For this review, take the finished solid that the model builds, in its own axes (mm). A direction names the side the tool comes from. Give positions to 0.01 mm unless a question says otherwise; leave off trailing zeros. Loops run counter-clockwise (first coordinate to the right, second up) from the corner with the lowest first, then second, coordinate; pieces in that order, holes last. Notation, with made-up numbers: (69.5, 73) - (121.5, 73) arc R18 ccw to (121.5, 94) - close; hole circle Ø4 at (62.25, 69.25). An arc over 180 degrees is marked (long way). Put each result on its own line as item: value.
from build123d import *

# Parameters (mm, degrees)
F1_DEPTH = 4
F3_DEPTH = 0.8


with BuildPart() as f1:
    # F0 (on Top) → F1 (new body)
    with BuildSketch(Plane.XY):
        Polygon((-9.1288570138, -20.6640837675), (-18.5707826287, -20.6640837675), (-18.5707826287, -32.6640837675), (6.4292173713, -32.6640837675), (6.4292173713, -20.6640837675), (-8.1288570138, -20.6640837675), (-11.2707826287, -22.8640837675), (4.2292173713, -22.8640837675), (4.2292173713, -30.4640837675), (-16.3707826287, -30.4640837675), (-16.3707826287, -22.8640837675), (-12.2707826287, -22.8640837675), align=None)
    extrude(amount=F1_DEPTH)

    # F2 (on face) → F3 (join)
    with BuildSketch(Plane.XY.offset(4)):
        with BuildLine():
            ThreePointArc((-7.2837039026, -27.5826807615), (-9.0353563223, -29.6788503531), (-11.6517702118, -30.4640837675))
            Line((-11.6517702118, -30.4640837675), (4.2292173713, -30.4640837675))
            Line((4.2292173713, -30.4640837675), (4.2292173713, -25.1570476435))
            Line((4.2292173713, -25.1570476435), (-3.6065624964, -25.1570476435))
            ThreePointArc((-3.6065624964, -25.1570476435), (-5.8091215163, -25.8180756813), (-7.2837039026, -27.5826807615))
        make_face()
    extrude(amount=-F3_DEPTH)


solid = f1.part
1) For faces 4 (the face through (-16.371, -27, 2)), 5 (the face through (-2, -28, 3.2)), 6 (the face through (-1, -20.664, 2)), list the 3-axis set-ups (+Z, -Z, +X, -X, +Y, -Y) from which the entire face can be reached by the end or side of a thin tool; tool diameter is ignored.
Geometry check:
face 4: +Z, -Z
face 5: -Z
face 6: +Z, -Z, +X, -X, +Y
2) Take a section at B-B on y = -24. State the section outline as (x, z) points, and give its area (3 significant figures).
Geometry check:
outline: (-18.57, 0) - (-16.37, 0) - (-16.37, 4) - (-18.57, 4) - close; (4.23, 0) - (6.43, 0) - (6.43, 4) - (4.23, 4) - close
area: 17.6 mm²
3) Take a section at C-C on x = -14. State the section outline as (y, z) points, and give its area (3 significant figures).
Geometry check:
outline: (-32.66, 0) - (-30.46, 0) - (-30.46, 4) - (-32.66, 4) - close; (-22.86, 0) - (-20.66, 0) - (-20.66, 4) - (-22.86, 4) - close
area: 17.6 mm²
4) Insertion check: pin 1 Ø4 at (x, y) = (-0.5, -26.5) entering from -Z. The pin has a flat end and moves straight along its axis. Give the tip position at first contact, or say it passes through.
Geometry check:
pin 1: stops at z = 3.2
5) Take a section at A-A on x = 0.75. State the section outline as (y, z) points.
Geometry check:
outline: (-32.66, 0) - (-30.46, 0) - (-30.46, 3.2) - (-25.16, 3.2) - (-25.16, 4) - (-32.66, 4) - close; (-22.86, 0) - (-20.66, 0) - (-20.66, 4) - (-22.86, 4) - close
6) Wall thickness on line 1 (X direction, y = -26, z = 1.4); line 2 (Y direction, x = -0.25, z = 3.75); line 3 (Y direction, x = -5.25, z = 2.2): over which ranges is each line inside the solid? List them lowest first.
Geometry check:
line 1: x = -18.57 to -16.37, 4.23 to 6.43
line 2: y = -32.66 to -25.16, -22.86 to -20.66
line 3: y = -32.66 to -30.46, -22.86 to -20.66
7) Draft analysis for pull direction Y (two halves, no side actions). For faces 1 (the face through (-6, -30.464, 2)), 2 (the face through (-6, -31, 0)), 3 (the face through (-6, -32.664, 2)), state which applies: pulls with the +Y half, pulls with the -Y half, needs draft (parallel to the pull), parting line crosses it, or undercut.
Geometry check:
face 1: undercut
face 2: needs draft
face 3: pulls with the -Y half
8) Take a section at D-D on z = 1.95. State the section outline as (x, y) points.
Geometry check:
outline: (-18.57, -32.66) - (6.43, -32.66) - (6.43, -20.66) - (-8.13, -20.66) - (-11.27, -22.86) - (4.23, -22.86) - (4.23, -30.46) - (-16.37, -30.46) - (-16.37, -22.86) - (-12.27, -22.86) - (-9.13, -20.66) - (-18.57, -20.66) - close
